Part model, mm, in its own coordinate system. A direction names the side the tool comes from. Coordinates: 2 decimals unless noted, no trailing zeros. Write each loop counter-clockwise with the first axis right and the second up, starting at its lowest first coordinate (ties: lowest second). Pieces come first, ordered by that corner, then holes. Notation, with made-up numbers: M -9.5,-8.5 L 9.5,-8.5 A10 cw 9.5,10.5 Z; hole C 36,18 d6. An arc over 180 degrees is marked long. Use a Markdown table: item, result. Add a question column.
Q1. Slice it at B-B on z = -34. Write the cut outline in (x, y), then the cut area to 3 significant figures.
Q2. Slice it at A-A on x = 118.5. Write the cut outline in (y, z).
Q3. Pin check, flat tips, straight feed: pin 1 Ø0.7 at (x, y) = (4.5, 1112.5) entering from -Z; pin 2 Ø0.7 at (y, z) = (1112.5, -52.5) entering from +X; pin 3 Ø0.7 at (y, z) = (1112.5, 51.5) entering from -X; pin 4 Ø12 at (x, z) = (-113.5, -106.5) entering from -Y. Stop position of each tip, or through.
Q4. Mould opens along Y. For faces 4 (the flat face through (197.79, 915.38, 186.7)), 5 (the flat face through (-3, 549, -236)), 6 (the flat face through (3, 0, 3)) say: released by +Y, released by -Y, zero draft, split by the parting line, or undercut.
Q5. Slice it at C-C on y = 816.5. Write the cut outline in (x, z).
Q6. Tool access for faces 1 (the flat face through (-184.205, 911, -33)), 2 (the flat face through (-3, 1111.55, -3)), 3 (the flat face through (3, 306, 236)): list every direction of +Z, -Z, +X, -X, +Y, -Y with a clear straight run to the whole face (end or side of a thin tool).
Q7. Wall check: L1, parallel to X at y = 971, z = -145.5; L2, parallel to Y at x = -1, z = -183; L3, parallel to Z at x = 172, y = 786. Give the ranges that are in metal, low to high. Write a range as from..to.
Autodesk Inventor part; units mm, degrees
ref_plane "YZ Plane" through (0, 0, 0) normal (1, 0, 0) x (0, 1, 0)
ref_plane "XZ Plane" through (0, 0, 0) normal (0, 1, 0) x (-1, 0, 0)
ref_plane "XY Plane" through (0, 0, 0) normal (0, 0, 1) x (1, 0, 0)
sketch "スケッチ1" plane through (0, 0, 0) normal (0, 1, 0) x (-1, 0, 0)
  line L0 (241, -236) -> (-241, -236)
  line L1 (-241, -236) -> (-241, 236)
  line L2 (-241, 236) -> (241, 236)
  line L3 (241, 236) -> (241, -236)
  line L4 (241, -236) -> (-241, 236) construction
  line L5 (-241, -236) -> (241, 236) construction
  point P0 (0, 0)
  dimension "d0" = 482
  dimension "d1" = 472
extrude "押し出し1" add sketch "スケッチ1" along normal blind 1113
fillet "フィレット1" radius 10 12 edges at (241, 1113, 0) (0, 1113, -236) (-241, 1113, 0) (0, 1113, 236) (-241, 556.5, 236) (241, 556.5, 236) (241, 556.5, -236) (-241, 556.5, -236) (0, 0, 236) (-241, 0, 0) (0, 0, -236) (241, 0, 0)
sketch "スケッチ2" plane through (0, 1113, 0) normal (0, 1, 0) x (1, 0, 0)
  line L0 (-212, -205) -> (212, -205)
  line L1 (212, -205) -> (212, 205)
  line L2 (212, 205) -> (-212, 205)
  line L3 (-212, 205) -> (-212, -205)
  line L4 (-212, -205) -> (212, 205) construction
  line L5 (212, -205) -> (-212, 205) construction
  point P0 (0, 0)
  dimension "d5" = 424
  dimension "d6" = 410
extrude "押し出し2" cut sketch "スケッチ2" against normal blind 1.45
sketch "スケッチ3" plane through (-231, 1103, 236) normal (0, 0, 1) x (1, 0, 0)
  line L0 (20, -20) -> (442, -20)
  line L1 (442, -20) -> (442, -360)
  line L2 (442, -360) -> (20, -360)
  line L3 (20, -360) -> (20, -20)
  point P0 (231, -1103)
  dimension "d9" = 422
  dimension "d10" = 340
extrude "押し出し3" cut sketch "スケッチ3" against normal blind 100
draft "面の勾配1" angle 15 pull direction (0, 0, 1) faces at (70.3333, 743, 202.6667) fixed edges at (0, 743, 236)
draft "面の勾配2" angle 15 pull direction (0, 0, 1) faces at (-211, 865.265, 202.6667) fixed edges at (-211, 913, 236)
draft "面の勾配3" angle 15 pull direction (0, 0, 1) faces at (-61.4017, 1083, 202.6667) fixed edges at (0, 1083, 236)
draft "面の勾配4" angle 15 pull direction (0, 0, 1) faces at (211, 865.265, 202.6667) fixed edges at (211, 913, 236)
sketch "スケッチ4" plane through (-231, 1103, 136) normal (0, 0, 1) x (1, 0, 0)
  line L0 (46.7949, -46.7949) -> (415.2051, -46.7949)
  line L1 (415.2051, -46.7949) -> (415.2051, -333.2051)
  line L2 (415.2051, -333.2051) -> (46.7949, -333.2051)
  line L3 (46.7949, -333.2051) -> (46.7949, -46.7949)
  point P0 (231, -1103)
extrude "押し出し4" cut sketch "スケッチ4" against normal blind 343
properties part number "box"
Recorded:
| question | item | result |
|---|---|---|
| 1 | outline | M -241,10 A10 ccw -231,0 L 231,0 A10 ccw 241,10 L 241,1103 A10 ccw 231,1113 L 212,1113 L 212,1111.55 L -212,1111.55 L -212,1113 L -231,1113 A10 ccw -241,1103 Z; hole M -184.21,769.79 L 184.21,769.79 L 184.21,1056.21 L -184.21,1056.21 Z |
| 1 | area | 430,000 mm² |
| 2 | outline | M 0,-226 A10 ccw 10,-236 L 1103,-236 A10 ccw 1113,-226 L 1113,-205 L 1111.55,-205 L 1111.55,205 L 1113,205 L 1113,226 A10 ccw 1103,236 L 1083,236 L 1056.21,136 L 1056.21,-207 L 769.79,-207 L 769.79,136 L 743,236 L 10,236 A10 ccw 0,226 Z |
| 3 | pin 1 | z = -230.03 |
| 3 | pin 2 | x = 235.03 |
| 3 | pin 3 | x = -235.03 |
| 3 | pin 4 | y = 0 |
| 4 | face 4 | undercut |
| 4 | face 5 | zero draft |
| 4 | face 6 | released by -Y |
| 5 | outline | M -241,-226 A10 ccw -231,-236 L 231,-236 A10 ccw 241,-226 L 241,226 A10 ccw 231,236 L 211,236 L 184.21,136 L 184.21,-207 L -184.21,-207 L -184.21,136 L -211,236 L -231,236 A10 ccw -241,226 Z |
| 6 | face 1 | +Z |
| 6 | face 2 | +Y |
| 6 | face 3 | +Z, +X, -X, +Y, -Y |
| 7 | L1 | -241..-184.21, 184.21..241 |
| 7 | L2 | 0..769.79, 1056.21..1111.55 |
| 7 | L3 | -236..-207 |
